```python
from build123d import *

# Parameters (mm, degrees)
SKETCH_1_R      = 3.4
SKETCH_1_W      = 5
SKETCH_1_H      = 5
EXTRUDE_1_DEPTH = 280


with BuildPart() as part:
    # 草图1 → 凸台-拉伸1 (new body)
    with BuildSketch(Plane(origin=(0, 0, 0), x_dir=(0, 0, -1), z_dir=(1, 0, 0))):
        Polygon((0, 6), (4.585786438, 6), (10.718811909, 12.133025471), (11, 13), (11, 18), (5.1, 18), (5.1, 20), (20, 20), (20, 5.1), (18, 5.1), (18, 11), (13, 11), (12.133025471, 10.718811909), (6, 4.585786438), (6, 0), (6, -4.585786438), (12.133025471, -10.718811909), (13, -11), (18, -11), (18, -5.1), (20, -5.1), (20, -20), (5.1, -20), (5.1, -18), (11, -18), (11, -13), (10.718811909, -12.133025471), (4.585786438, -6), (0, -6), (-4.585786438, -6), (-10.718811909, -12.133025471), (-11, -13), (-11, -18), (-5.1, -18), (-5.1, -20), (-20, -20), (-20, -5.1), (-18, -5.1), (-18, -11), (-13, -11), (-12.133025471, -10.718811909), (-6, -4.585786438), (-6, 0), (-6, 4.585786438), (-12.133025471, 10.718811909), (-13, 11), (-18, 11), (-18, 5.1), (-20, 5.1), (-20, 20), (-5.1, 20), (-5.1, 18), (-11, 18), (-11, 13), (-10.718811909, 12.133025471), (-4.585786438, 6), align=None)
        Circle(SKETCH_1_R, mode=Mode.SUBTRACT)
        with Locations((15.5, -15.5)):
            Rectangle(SKETCH_1_W, SKETCH_1_H, mode=Mode.SUBTRACT)
        with Locations((15.5, 15.5)):
            Rectangle(SKETCH_1_W, SKETCH_1_H, mode=Mode.SUBTRACT)
        with Locations((-15.5, -15.5)):
            Rectangle(SKETCH_1_W, SKETCH_1_H, mode=Mode.SUBTRACT)
        with Locations((-15.5, 15.5)):
            Rectangle(SKETCH_1_W, SKETCH_1_H, mode=Mode.SUBTRACT)
    extrude(amount=EXTRUDE_1_DEPTH)


solid = part.part
```
Verification items for the finished model (mm, model axes). A direction names the side the tool comes from. Coordinates: 2 decimals unless noted, no trailing zeros. Loops run counter-clockwise (first coordinate to the right, second up) from the corner with the lowest first, then second, coordinate; pieces in that order, holes last. Notation, with made-up numbers: (15, -22.75) - (32, -22.75) arc R31 ccw to (32, 7.25) - close; hole circle Ø3 at (-21.5, 16). An arc over 180 degrees is marked (long way). Return JSON: item names as keys, results as strings.
1. Go/stop test with flat-tipped pins: pin 1 (10 mm diameter, centred on x = 194.5, z = 0.5, fed in from +Y); pin 2 (3 mm diameter, centred on x = 195, z = -0.5, fed in from -Y). Record where each tip stops, or that it passes through.
Established:
{"pin 1": "stops at y = 20", "pin 2": "stops at y = -6"}
2. Section check A-A, the plane y = 0. Record the boundary of the cut face in (x, z).
Established:
{"outline": "(0, -6) - (280, -6) - (280, -3.4) - (0, -3.4) - close; (0, 3.4) - (280, 3.4) - (280, 6) - (0, 6) - close"}
3. Thickness scan on L1, parallel to Z at x = 24, y = -15; L2, parallel to Y at x = 165.5, z = 0. Record the ranges inside material, lowest first.
Established:
{"L1": "z = -20 to -18, -13 to -11, 11 to 13, 18 to 20", "L2": "y = -6 to -3.4, 3.4 to 6"}
4. Section check C-C, the plane x = 34.5. Count the separate pieces of the cut face and the enclosed holes in it, then the cut area to 3 significant figures.
Established:
{"separate pieces": "1", "enclosed holes": "5", "area": "491 mm2"}
5. Mould release check, pull along Y, two halves, no side actions. Record for faces 1 (the flat face through (138, -6, 0)), 2 (the flat face through (138, 11, -16)), 3 (the flat face through (138, 13, -20)): +Y half, -Y half, draft (parallel to the pull), parting line (faces both ways), or undercut.
Established:
{"face 1": "-Y half", "face 2": "undercut", "face 3": "draft"}
6. Tool access check on faces 4 (the flat face through (138, -12, -20)), 5 (the flat face through (138, 15, 18)), 6 (the flat face through (138, 6, 0)). Record the directions out of +Z, -Z, +X, -X, +Y, -Y that give a thin tool (end or side, any length) a straight path to the whole face; none if there is none.
Established:
{"face 4": "-Z, +X, -X, +Y, -Y", "face 5": "+X, -X", "face 6": "+X, -X, +Y"}
